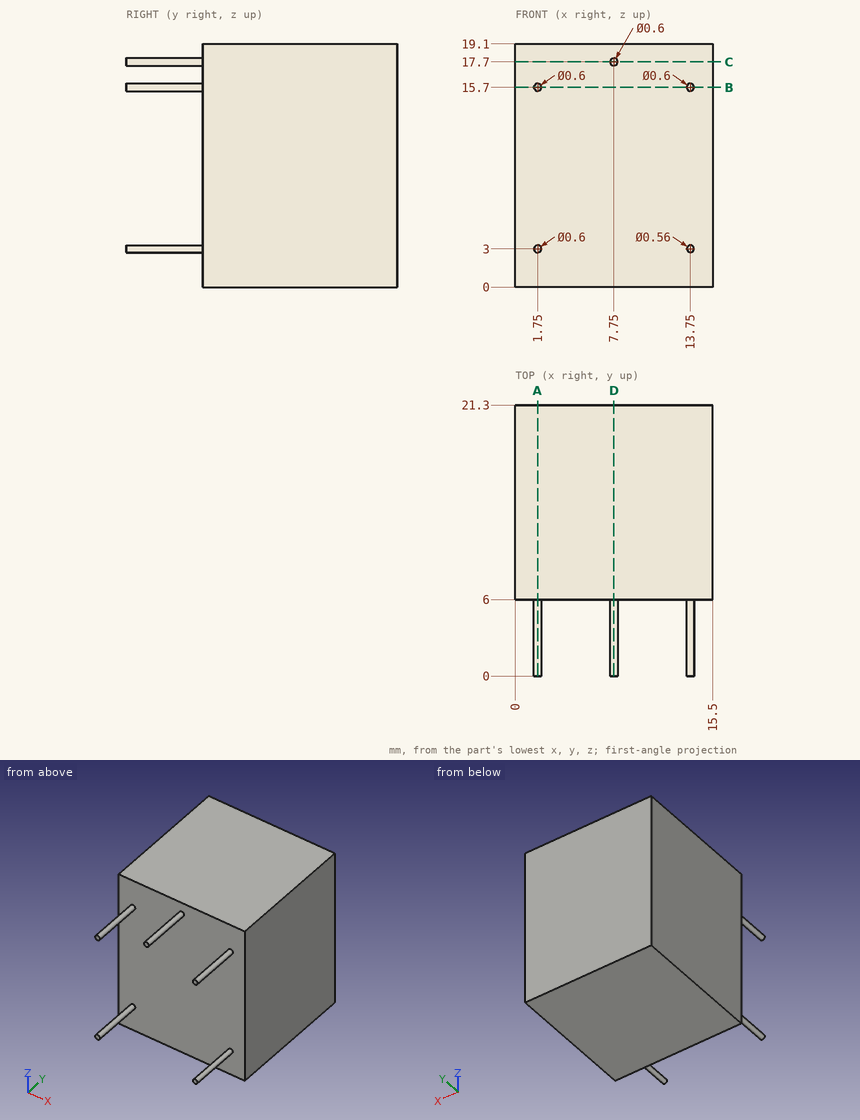
Could you check a few things on this drawing? It's one solid part, dimensions in mm from its lowest x, y, z. Give positions to 0.01 mm unless a question says otherwise; leave off trailing zeros. Loops run counter-clockwise (first coordinate to the right, second up) from the corner with the lowest first, then second, coordinate; pieces in that order, holes last. Notation, with made-up numbers: (25.25, 29.5) -> (32.25, 29.5) arc R19 cw to (32.25, 62.5) -> close; hole circle Ø6 at (-1, 14.25). An arc over 180 degrees is marked (long way). Answer as CSV lines item,"result". Start each with the question number.
(1) If we section it at A-A on x = 1.75: Write out the boundary of the cut face in (y, z).
(2) If we section it at B-B on z = 15.7: Write out the boundary of the cut face in (x, y).
(3) I need wall thicknesses on probe 1 along Y at (x, z) = (4, 16). Which ranges of the line are inside material? Lowest first, please.
(4) If we section it at D-D on x = 7.75: Write out the boundary of the cut face in (y, z), then the cut area to 3 significant figures.
(5) I'm going to push a flat-ended pin straight in: pin 1 Ø4.5 at (x, z) = (10.5, 9) entering from -Y. Where does the tip first touch, or does it pass through?
(6) If we section it at C-C on z = 17.7: Write out the boundary of the cut face in (x, y), then the cut area to 3 significant figures.
Computed:
1,outline,"(0, 2.7) -> (6, 2.7) -> (6, 0) -> (21.3, 0) -> (21.3, 19.1) -> (6, 19.1) -> (6, 16) -> (0, 16) -> (0, 15.4) -> (6, 15.4) -> (6, 3.3) -> (0, 3.3) -> close"
2,outline,"(0, 6) -> (1.45, 6) -> (1.45, 0) -> (2.05, 0) -> (2.05, 6) -> (13.45, 6) -> (13.45, 0) -> (14.05, 0) -> (14.05, 6) -> (15.5, 6) -> (15.5, 21.3) -> (0, 21.3) -> close"
3,probe 1,"y = 6 to 21.3"
4,outline,"(0, 17.4) -> (6, 17.4) -> (6, 0) -> (21.3, 0) -> (21.3, 19.1) -> (6, 19.1) -> (6, 18) -> (0, 18) -> close"
4,area,"296 mm2"
5,pin 1,"stops at y = 6"
6,outline,"(0, 6) -> (7.45, 6) -> (7.45, 0) -> (8.05, 0) -> (8.05, 6) -> (15.5, 6) -> (15.5, 21.3) -> (0, 21.3) -> close"
6,area,"241 mm2"
